Input: dimensioned drawing with shaded views. Units: mm. Origin: part minimum x, y, z. A direction names the side the tool comes from. Round coordinates to 2 decimals unless told otherwise and drop trailing zeros. Loops run counter-clockwise (first coordinate to the right, second up) from the corner with the lowest first, then second, coordinate; pieces in that order, holes last. Notation, with made-up numbers: M 20.5,29.25 L 78.5,29.25 A16 cw 78.5,38.25 Z; hole C -2.5,-20 d4. An arc over 180 degrees is marked long. Return JSON: item names as keys, results as strings.
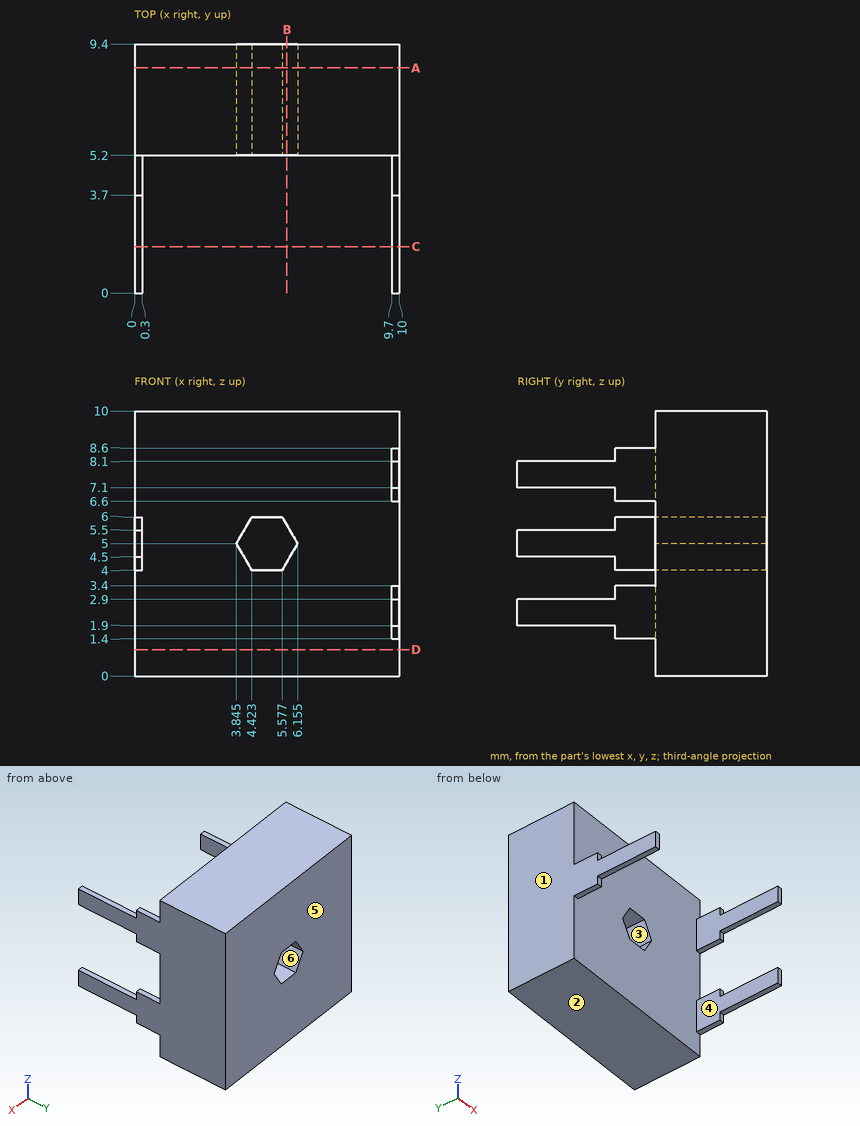
Q1. Section query D-D (z = 1). Output: boundary loops of the cut face in (x, y).
Determined:
{"outline": "M 0,5.2 L 10,5.2 L 10,9.4 L 0,9.4 Z"}
Q2. Section query B-B (x = 5.75). Output: boundary loops of the cut face in (y, z), plus the area to 3 significant figures.
Determined:
{"outline": "M 5.2,0 L 9.4,0 L 9.4,4.3 L 5.2,4.3 Z; M 5.2,5.7 L 9.4,5.7 L 9.4,10 L 5.2,10 Z", "area": "36.1 mm^2"}
Q3. Material intervals for L1, parallel to Z at x = 5.5, y = 7.75; L2, parallel to Y at x = 1.75, z = 6.5, sorted ascending.
Determined:
{"L1": "z = 0 to 4, 6 to 10", "L2": "y = 5.2 to 9.4"}
Q4. Section query C-C (y = 1.75). Output: boundary loops of the cut face in (x, z).
Determined:
{"outline": "M 0,4.5 L 0.3,4.5 L 0.3,5.5 L 0,5.5 Z; M 9.7,1.9 L 10,1.9 L 10,2.9 L 9.7,2.9 Z; M 9.7,7.1 L 10,7.1 L 10,8.1 L 9.7,8.1 Z"}
Q5. Pull-direction query (X, two-part tool) for the marked faces 1, 2 and 3; classes: pulls with the +X half, pulls with the -X half, needs draft (parallel to the pull), parting line crosses it, or undercut.
Determined:
{"face 1": "pulls with the -X half", "face 2": "needs draft", "face 3": "undercut"}
Q6. Section query A-A (y = 8.5). Output: boundary loops of the cut face in (x, z) (1 decimal).
Determined:
{"outline": "M 0,0 L 10,0 L 10,10 L 0,10 Z; hole M 3.8,5 L 4.4,4 L 5.6,4 L 6.2,5 L 5.6,6 L 4.4,6 Z"}
Q7. Reachability of the marked faces 4, 5 and 6 from +Z, -Z, +X, -X, +Y, -Y: full face, straight path, thin tool, end or side. Return the list, or none.
Determined:
{"face 4": "+Z, -Z, -X, -Y", "face 5": "+Z, -Z, +X, -X, +Y", "face 6": "+Y, -Y"}
Q8. Pin query (flat end, axial travel): pin 1 (5 mm diameter, centred on x = 3.5, z = 7, fed in from -Y). Return the tip coordinate at first contact, or that it passes through.
Determined:
{"pin 1": "stops at y = 5.2"}
